Check sheet for the drawn part. Datum: minimum x, y, z corner. Units: mm. A direction names the side the tool comes from. Coordinates: 2 decimals unless noted, no trailing zeros. Loops run counter-clockwise (first coordinate to the right, second up) from the corner with the lowest first, then second, coordinate; pieces in that order, holes last.
Q1. Material ranges on probe 1 along Y at (x, z) = (13, 5.5); probe 2 along X at (y, z) = (26.5, 18.5); probe 3 along Z at (x, y) = (28, 17) (1 decimal), recorded low to high.
Q2. Sectioned sample at C-C (x = 18). Enter the section's corners in (y, z).
Q3. Go/stop test with flat-tipped pins: P1, Ø2, axis at x = 30, y = 27.5, coming from the +Z side; P2, Ø5, axis at x = 4, z = 11, coming from the -Y side; P3, Ø4, axis at y = 17.5, z = 12.5, coming from the -X side. Record where each tip stops, or that it passes through.
Q4. Access from +Z, -Z, +X, -X, +Y, -Y to the whole of each face (thin tool, end or side, straight path). Record for the marked faces 1 and 2.
Q5. Sectioned sample at D-D (z = 32.5). Enter the section's corners in (x, y) (1 decimal).
Q6. Sectioned sample at B-B (y = 16). Enter the section's corners in (x, z), then the cut area to 3 significant figures.
Q7. Sectioned sample at A-A (z = 26). Enter the section's corners in (x, y) (1 decimal), then the cut area to 3 significant figures.
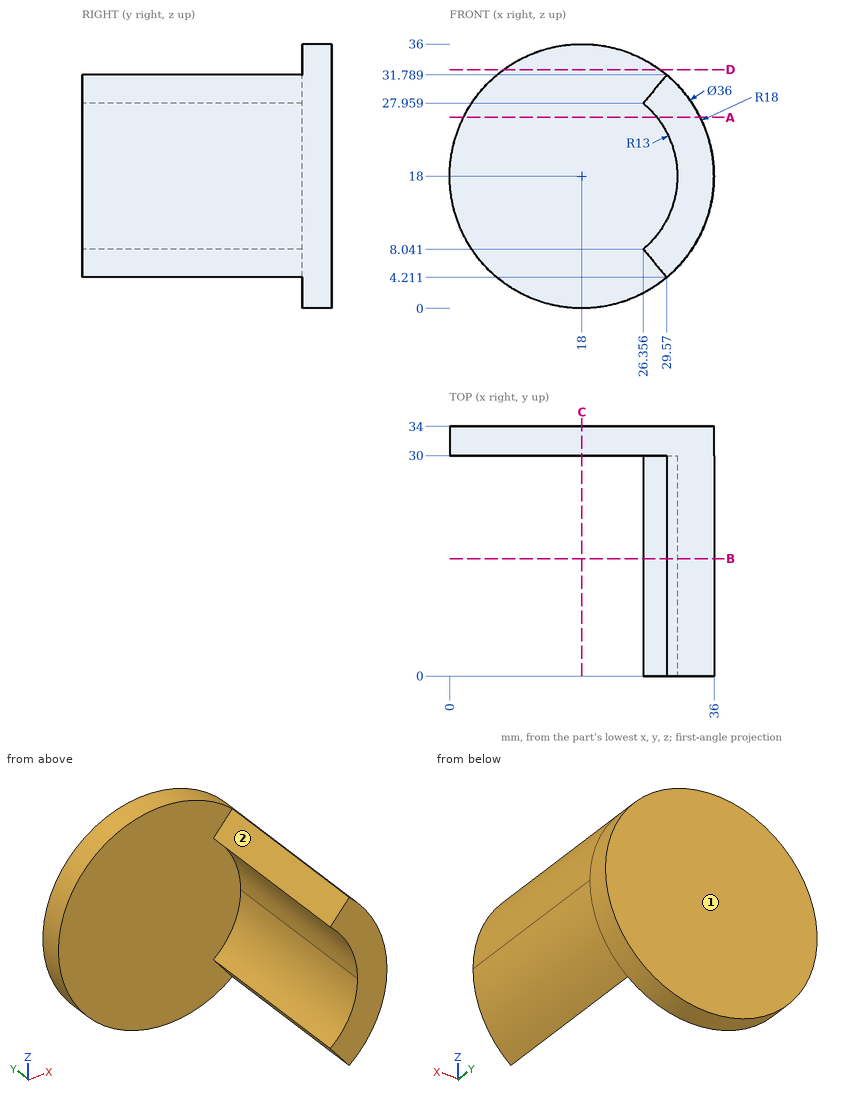
Geometry check:
1. probe 1: y = 30 to 34
1. probe 2: x = 30.99 to 35.99
1. probe 3: z = 6.1 to 9.7, 26.3 to 29.9
2. outline: (30, 0) - (34, 0) - (34, 36) - (30, 36) - close
3. P1: stops at z = 31.79
3. P2: stops at y = 30
3. P3: stops at x = 28.62
4. face 1: +Z, -Z, +X, -X, +Y
4. face 2: +Z, -X, -Y
5. outline: (7.3, 30) - (28.7, 30) - (28.7, 34) - (7.3, 34) - close
6. outline: (26.36, 8.04) - (29.57, 4.21) arc R18 ccw to (29.57, 31.79) - (26.36, 27.96) arc R13 cw to start
6. area: 135 mm2
7. outline: (1.9, 30) - (28.2, 30) - (28.2, 0) - (34.1, 0) - (34.1, 34) - (1.9, 34) - close
7. area: 305 mm2
